The model under review builds one solid part; all positions refer to its coordinate system, in mm. A direction names the side the tool comes from. Coordinates: 2 decimals unless noted, no trailing zeros. Write each loop counter-clockwise with the first axis right and the second up, starting at its lowest first coordinate (ties: lowest second). Pieces come first, ordered by that corner, then holes. Notation, with made-up numbers: (-7.75, 76) - (17.25, 76) arc R22 cw to (17.25, 90) - close; hole circle Ø7 at (46, -21). An arc over 180 degrees is marked (long way). Put each result on its own line as item: value. Start each with the question number.
Item 1: To check wall thickness, follow L1, parallel to Y at x = -0.05, z = -13.5; L2, parallel to Y at x = 0, z = -15.55; L3, parallel to Z at x = 2, y = -2. State the ranges of each line that lie inside material, in increasing order. Write a range as [from, to].
Item 2: Machinability: for faces 5 (the face through (0.75, -6, -9)), 6 (the face through (0, -3, -9)), 7 (the face through (-0.75, -6, -9)), which of the approach directions +Z, -Z, +X, -X, +Y, -Y give a long, thin tool a straight path to every point of the face, cutting with its end or side? Answer none if there is none.
Item 3: For pin 1 (2.5 mm diameter, centred on x = 0, y = 0, fed in from -Z); pin 2 (2.5 mm diameter, centred on y = -6, z = -13.5, fed in from +X); pin 3 (2 mm diameter, centred on x = -1, z = -11, fed in from +Y); pin 4 (3 mm diameter, centred on y = -4.5, z = -13, fed in from -X), all flat-tipped, find the tip position at first contact; note any pin that passes through.
Item 4: Consider section A-A on z = -4. Give the boundary of the cut face in (x, y), then the cut area to 3 significant figures.
Item 5: Mouldability with a two-part tool opening along Y and no side actions: class faces 1 (the face through (0, 3, -2)), 2 (the face through (0, -2, -15)), 3 (the face through (0, -3, 0)), 4 (the face through (0.01, -5.97, -12.75)) as pulls with the +Y half, pulls with the -Y half, needs draft (parallel to the pull), parting line crosses it, or undercut.
Item 6: Consider section C-C on x = -1.15. Give the boundary of the cut face in (y, z).
Item 7: Consider section D-D on y = -6. Give the boundary of the cut face in (x, z).
Item 8: Consider section B-B on y = 0. Give the boundary of the cut face in (x, z).
```python
from build123d import *

# Parameters (mm, degrees)
SKETCH2_R           = 3
SKETCH2_R_2         = 2
SKETCH2_W           = 1.5
SKETCH2_H           = 6
BOSS_EXTRUDE4_DEPTH = 17.5
CUT_EXTRUDE3_START  = -5
SKETCH2_4_R         = 3
CUT_EXTRUDE3_DEPTH  = 7.5
SKETCH4_R           = 0.75
CUT_EXTRUDE6_DEPTH  = 10


with BuildPart() as part:
    # Sketch2 → Boss-Extrude4 (new body)
    # profile 1 of 2: a face of its own
    with BuildSketch(Plane.XY):
        Circle(SKETCH2_R)
        Circle(SKETCH2_R_2, mode=Mode.SUBTRACT)
    # profile 2 of 2: a face of its own
    with BuildSketch(Plane.XY):
        with Locations((0, -5.9)):
            Rectangle(SKETCH2_W, SKETCH2_H)
    extrude(amount=-BOSS_EXTRUDE4_DEPTH)

    # Sketch2_4 → Cut-Extrude3 (cut)
    with BuildSketch(Plane.XY.offset(CUT_EXTRUDE3_START)):
        Circle(SKETCH2_4_R)
    extrude(amount=-CUT_EXTRUDE3_DEPTH, mode=Mode.SUBTRACT)

    # Sketch4 → Cut-Extrude6 (cut)
    with BuildSketch(Plane(origin=(0.75, 0, 0), x_dir=(0, 0, -1), z_dir=(1, 0, 0))):
        with Locations((4, -6)):
            Circle(SKETCH4_R)
        with Locations((13.5, -6)):
            Circle(SKETCH4_R)
    extrude(amount=-CUT_EXTRUDE6_DEPTH, mode=Mode.SUBTRACT)


solid = part.part
```
Report:
1. L1: [-8.9, -6.75], [-5.25, -2], [2, 3]
1. L2: [-8.9, -2], [2, 3]
1. L3: [-17.5, -12.5], [-5, 0]
2. face 5: +Z, -Z, +X, -Y
2. face 6: +Y
2. face 7: +Z, -Z, -X, -Y
3. pin 1: through
3. pin 2: x = 0.75
3. pin 3: y = -2.9
3. pin 4: x = -0.75
4. outline: (-0.75, -8.9) - (0.75, -8.9) - (0.75, -6.75) - (-0.75, -6.75) - close; (-0.75, -5.25) - (0.75, -5.25) - (0.75, -2.9) arc R3 ccw (long way) to (-0.75, -2.9) - close; hole circle Ø4 at (0, 0)
4. area: 22.4 mm²
5. face 1: parting line crosses it
5. face 2: undercut
5. face 3: needs draft
5. face 4: undercut
6. outline: (-2.77, -17.5) - (-1.64, -17.5) - (-1.64, -12.5) - (-2.77, -12.5) - close; (-2.77, -5) - (-1.64, -5) - (-1.64, 0) - (-2.77, 0) - close; (1.64, -17.5) - (2.77, -17.5) - (2.77, -12.5) - (1.64, -12.5) - close; (1.64, -5) - (2.77, -5) - (2.77, 0) - (1.64, 0) - close
7. outline: (-0.75, -17.5) - (0.75, -17.5) - (0.75, -14.25) - (-0.75, -14.25) - close; (-0.75, -12.75) - (0.75, -12.75) - (0.75, -4.75) - (-0.75, -4.75) - close; (-0.75, -3.25) - (0.75, -3.25) - (0.75, 0) - (-0.75, 0) - close
8. outline: (-3, -17.5) - (-2, -17.5) - (-2, -12.5) - (-3, -12.5) - close; (-3, -5) - (-2, -5) - (-2, 0) - (-3, 0) - close; (2, -17.5) - (3, -17.5) - (3, -12.5) - (2, -12.5) - close; (2, -5) - (3, -5) - (3, 0) - (2, 0) - close
